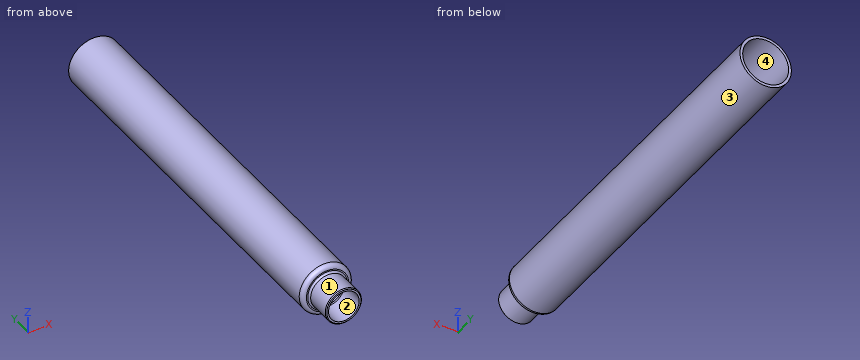
```python
from build123d import *

# Parameters (mm, degrees)
CHANFREIN1_SIZE = 0.5


with BuildPart() as part:
    # Esquisse1 → Révolution1 (revolve)
    with BuildSketch(Plane.XY, mode=Mode.PRIVATE) as r_volution1_sk:
        with BuildLine():
            Line((8.5, -15), (8.5, -1))
            ThreePointArc((8.5, -1), (9.232233047, 0.767766953), (11, 1.5))
            Line((11, 1.5), (11.75, 1.5))
            ThreePointArc((11.75, 1.5), (12.457106781, 1.792893219), (12.75, 2.5))
            Line((12.75, 2.5), (12.75, 215))
            Line((12.75, 215), (14.25, 215))
            Line((14.25, 215), (14.25, 2.5))
            ThreePointArc((14.25, 2.5), (13.517766953, 0.732233047), (11.75, 0))
            Line((11.75, 0), (11, 0))
            ThreePointArc((11, 0), (10.292893219, -0.292893219), (10, -1))
            Line((10, -1), (10, -15))
            Line((10, -15), (8.5, -15))
        make_face()
    revolve(r_volution1_sk.sketch.rotate(Axis((0, 34.901303155, 0), (0, -1, 0)), 90), axis=Axis((0, 34.901303155, 0), (0, -1, 0)))  # turned: the seam where the file's is

    # Chanfrein1
    chanfrein1_edges = [part.edges().sort_by_distance(p)[0] for p in [
        (0, -15, -10),
    ]]
    chamfer(chanfrein1_edges, length=CHANFREIN1_SIZE)


solid = part.part
```
Part model, mm, in its own coordinate system. Face numbers are marked on the shaded views. A direction names the side the tool comes from. Round coordinates to 2 decimals unless told otherwise and drop trailing zeros. Write each loop counter-clockwise with the first axis right and the second up, starting at its lowest first coordinate (ties: lowest second). Pieces come first, ordered by that corner, then holes.
Item 1: Cut at A-A, the plane z = 0. Give the cut face in (x, y), plus the area to 3 significant figures.
Results:
outline: (-14.25, 2.5) arc R2.5 ccw to (-11.75, 0) - (-11, 0) arc R1 cw to (-10, -1) - (-10, -14.5) - (-9.5, -15) - (-8.5, -15) - (-8.5, -1) arc R2.5 ccw to (-11, 1.5) - (-11.75, 1.5) arc R1 cw to (-12.75, 2.5) - (-12.75, 215) - (-14.25, 215) - close; (8.5, -15) - (9.5, -15) - (10, -14.5) - (10, -1) arc R1 cw to (11, 0) - (11.75, 0) arc R2.5 ccw to (14.25, 2.5) - (14.25, 215) - (12.75, 215) - (12.75, 2.5) arc R1 cw to (11.75, 1.5) - (11, 1.5) arc R2.5 ccw to (8.5, -1) - close
area: 698 mm2
Item 2: Cut at C-C, the plane y = 180. Give the cut face in (x, z), plus the area to 3 significant figures.
Results:
outline: circle Ø28.5 at (0, 0); hole circle Ø25.5 at (0, 0)
area: 127 mm2
Item 3: Two-plate mould, pull along X, no slides. Class the marked faces 1 and 2: +X half, -X half, draft (parallel to the pull), parting line (faces both ways), or undercut.
Results:
face 1: parting line
face 2: undercut
Item 4: Drop flat-ended pins along their axis: pin 1 Ø8 at (x, z) = (0.5, -2.5) entering from -Y; pin 2 Ø10 at (y, z) = (147, -9) entering from -X; pin 3 Ø4 at (y, z) = (92, -4) entering from +X; pin 4 Ø12 at (x, y) = (8, 73.5) entering from +Z. Give the stop position or say it passes through.
Results:
pin 1: passes through
pin 2: stops at x = -13.68
pin 3: stops at x = 14.11
pin 4: stops at z = 14.11
Item 5: Cut at B-B, the plane x = 0. Give the cut face in (y, z).
Results:
outline: (-15, -9.5) - (-14.5, -10) - (-1, -10) arc R1 cw to (0, -11) - (0, -11.75) arc R2.5 ccw to (2.5, -14.25) - (215, -14.25) - (215, -12.75) - (2.5, -12.75) arc R1 cw to (1.5, -11.75) - (1.5, -11) arc R2.5 ccw to (-1, -8.5) - (-15, -8.5) - close; (-15, 8.5) - (-1, 8.5) arc R2.5 ccw to (1.5, 11) - (1.5, 11.75) arc R1 cw to (2.5, 12.75) - (215, 12.75) - (215, 14.25) - (2.5, 14.25) arc R2.5 ccw to (0, 11.75) - (0, 11) arc R1 cw to (-1, 10) - (-14.5, 10) - (-15, 9.5) - close
Item 6: Probe L1, parallel to X at y = 107.5, z = 0; L2, parallel to X at y = -8.5, z = 0; L3, parallel to Z at x = -4, y = 178. List the from-to ranges inside material, lowest first.
Results:
L1: x = -14.25 to -12.75, 12.75 to 14.25
L2: x = -10 to -8.5, 8.5 to 10
L3: z = -13.68 to -12.11, 12.11 to 13.68
Item 7: Which spindle directions (+Z, -Z, +X, -X, +Y, -Y) get a long thin tool onto all of the face, cutting with end or side? Do the marked faces 3 and 4. Say none if no direction does.
Results:
face 3: +Y, -Y
face 4: +Y
